Autodesk Fusion 360 part; units mm, degrees
sketch "Sketch1" plane through (0, 0, 0) normal (0, 0, 1) x (1, 0, 0)
  line L0 (-17.3001, 65.9212) -> (152.6999, 65.9212)
  line L1 (152.6999, 65.9212) -> (152.6999, -74.0788)
  line L2 (152.6999, -74.0788) -> (-17.3001, -74.0788)
  line L3 (-17.3001, -74.0788) -> (-17.3001, 65.9212)
  dimension "d1" = 140
  dimension "d2" = 170
extrude "Extrude1" add sketch "Sketch1" along normal blind 5
sketch "Sketch6" plane through (0, 0, 5) normal (0, 0, 1) x (-1, 0, 0)
  line L0 (17.3001, 74.0788) -> (-152.6999, 74.0788)
  line L1 (-152.6999, 74.0788) -> (-152.6999, -65.9212)
  line L2 (-152.6999, -65.9212) -> (17.3001, -65.9212)
  line L3 (17.3001, -65.9212) -> (17.3001, 74.0788)
  line L4 (-2.6999, 54.0788) -> (-132.6999, 54.0788)
  line L5 (-132.6999, 54.0788) -> (-132.6999, -45.9212)
  line L6 (-132.6999, -45.9212) -> (-2.6999, -45.9212)
  line L7 (-2.6999, -45.9212) -> (-2.6999, 54.0788)
  line L8 (17.3001, 74.0788) -> (17.3001, -65.9212)
  line L9 (-152.6999, -65.9212) -> (-152.6999, 74.0788)
  line L10 (-152.6999, 74.0788) -> (17.3001, 74.0788)
  line L11 (17.3001, -65.9212) -> (-152.6999, -65.9212)
  line L12 (-2.6999, 54.0788) -> (-12.6999, 54.0788)
  line L13 (-12.6999, 54.0788) -> (-12.6999, 44.0788)
  line L14 (-12.6999, 44.0788) -> (-2.6999, 44.0788)
  line L15 (-2.6999, 44.0788) -> (-2.6999, 54.0788)
  line L16 (-2.6999, -45.9212) -> (-12.6999, -45.9212)
  line L17 (-12.6999, -45.9212) -> (-12.6999, -35.9212)
  line L18 (-12.6999, -35.9212) -> (-2.6999, -35.9212)
  line L19 (-2.6999, -35.9212) -> (-2.6999, -45.9212)
  line L20 (-132.6999, 54.0788) -> (-122.6999, 54.0788)
  line L21 (-122.6999, 54.0788) -> (-122.6999, 44.0788)
  line L22 (-122.6999, 44.0788) -> (-132.6999, 44.0788)
  line L23 (-132.6999, 44.0788) -> (-132.6999, 54.0788)
  line L24 (-132.6999, -45.9212) -> (-122.6999, -45.9212)
  line L25 (-122.6999, -45.9212) -> (-122.6999, -35.9212)
  line L26 (-122.6999, -35.9212) -> (-132.6999, -35.9212)
  line L27 (-132.6999, -35.9212) -> (-132.6999, -45.9212)
  line L28 (-62.6999, 54.0788) -> (-72.6999, 54.0788)
  line L29 (-72.6999, 54.0788) -> (-72.6999, 44.0788)
  line L30 (-72.6999, 44.0788) -> (-62.6999, 44.0788)
  line L31 (-62.6999, 44.0788) -> (-62.6999, 54.0788)
  line L32 (-62.6999, -45.9212) -> (-72.6999, -45.9212)
  line L33 (-72.6999, -45.9212) -> (-72.6999, -35.9212)
  line L34 (-72.6999, -35.9212) -> (-62.6999, -35.9212)
  line L35 (-62.6999, -35.9212) -> (-62.6999, -45.9212)
  line L36 (-22.6999, -25.9212) -> (-112.6999, -25.9212)
  line L37 (-112.6999, -25.9212) -> (-112.6999, 34.0788)
  line L38 (-112.6999, 34.0788) -> (-22.6999, 34.0788)
  line L39 (-22.6999, 34.0788) -> (-22.6999, -25.9212)
  dimension "d23" = 20
  dimension "d24" = 20
  dimension "d25" = 20
  dimension "d26" = 20
  dimension "d27" = 10
  dimension "d28" = 10
  dimension "d29" = 10
  dimension "d30" = 10
  dimension "d31" = 10
  dimension "d32" = 10
  dimension "d33" = 10
  dimension "d34" = 10
  dimension "d35" = 10
  dimension "d36" = 10
  dimension "d37" = 10
  dimension "d38" = 10
  dimension "d39" = 50
  dimension "d40" = 50
  dimension "d41" = 50
  dimension "d42" = 50
  dimension "d57" = 10
  dimension "d58" = 10
  dimension "d59" = 10
  dimension "d60" = 10
  dimension "d61" = 20
  dimension "d62" = 20
extrude "Extrude4" add sketch "Sketch6" along normal blind 105 contours L4 L7 L12 L13 L14 L15 | L4 L28 L29 L30 L31 | L6 L7 L16 L17 L18 L19 | L4 L5 L20 L21 L22 L23 | L6 L32 L33 L34 L35 | L5 L6 L24 L25 L26 L27
sketch "Sketch7" plane through (0, 0, 110) normal (0, 0, 1) x (-1, 0, 0)
  line L0 (-2.6999, 44.0788) -> (-2.6999, 54.0788)
  line L1 (-2.6999, 54.0788) -> (-12.6999, 54.0788)
  line L2 (-12.6999, 54.0788) -> (-12.6999, 44.0788)
  line L3 (-12.6999, 44.0788) -> (-2.6999, 44.0788)
  line L4 (-2.6999, 54.0788) -> (-132.6999, 54.0788)
  line L5 (-132.6999, 54.0788) -> (-132.6999, -45.9212)
  line L6 (-132.6999, -45.9212) -> (-2.6999, -45.9212)
  line L7 (-2.6999, -45.9212) -> (-2.6999, 54.0788)
  dimension "d45" = 130
  dimension "d46" = 100
extrude "Extrude5" add sketch "Sketch7" along normal blind 5
sketch "Sketch8" plane through (0, 0, 115) normal (0, 0, 1) x (-1, 0, 0)
  line L0 (-2.6999, -45.9212) -> (-2.6999, 54.0788)
  line L1 (-2.6999, 54.0788) -> (-132.6999, 54.0788)
  line L2 (-132.6999, 54.0788) -> (-132.6999, -45.9212)
  line L3 (-132.6999, -45.9212) -> (-2.6999, -45.9212)
  line L4 (-57.6999, -15.9212) -> (-77.6999, -15.9212)
  line L5 (-77.6999, -15.9212) -> (-77.6999, 24.0788)
  line L6 (-77.6999, 24.0788) -> (-57.6999, 24.0788)
  line L7 (-57.6999, 24.0788) -> (-57.6999, -15.9212)
  dimension "d49" = 40
  dimension "d50" = 20
  dimension "d51" = 55
  dimension "d52" = 55
  dimension "d53" = 30
  dimension "d54" = 30
extrude "Extrude6" add sketch "Sketch8" along normal blind 5 contours L4 L5 L6 L7
extrude "Extrude7" cut sketch "Sketch6" against normal blind 5 contours L36 L37 L38 L39
Geometry: final body of the model. Coordinates: model frame, mm. A direction names the side the tool comes from. Give positions to 0.01 mm unless a question says otherwise; leave off trailing zeros. Order: outer loops, then holes, each group sorted by start corner. A loop starts at its lowest first (then second) coordinate and runs counter-clockwise, first axis right, second up. Notation, with made-up numbers: (9.25, -0.75) -> (30.25, -0.75) arc R22 ccw to (30.25, 31.25) -> close; hole circle Ø11 at (27, -15.75). An arc over 180 degrees is marked (long way). Write each question's results on one line, items separated by ' | '. Start each with the question number.
1) Section D-D (y = -21.5). Return loops of the section in (x, z), then the cut area to 3 significant figures.
2) First-contact query: pin 1 (3 mm diameter, centred on y = 43, z = 105, fed in from -X); pin 2 (8 mm diameter, centred on y = 43, z = 53, fed in from +X); pin 3 (3 mm diameter, centred on x = 129, z = 50, fed in from +Y). Flat tips, straight axial feed; report the tip coordinate or a pass-through.
3) Section A-A (y = -37.5). Return loops of the section in (x, z), then the cut area to 3 significant figures.
4) Draft query along Z for faces 1 (the flat face through (72.7, -49, 57)), 2 (the flat face through (57.7, -4, 117)), 3 (the flat face through (67, 28, 0)), 4 (the flat face through (62.7, -49, 57)). Return one class per face: pulls with the +Z half, pulls with the -Z half, needs draft (parallel to the pull), parting line crosses it, or undercut.
5) Set-up query: faces 5 (the flat face through (132.7, -45, 68)), 6 (the flat face through (22.7, -4, 3)), 7 (the flat face through (68, 45.921, 64)). Return all of +Z, -Z, +X, -X, +Y, -Y with unobstructed straight access to the full face (end or side cutting, diameter ignored); none if empty.
6) Section B-B (z = 22). Return loops of the section in (x, y), then the cut area to 3 significant figures.
7) Section C-C (x = 17.5). Return loops of the section in (y, z), then the cut area to 3 significant figures.
8) Line query: line 1 (X direction, y = 45, z = 94.5); line 2 (Z direction, x = 103, y = -46); line 3 (Y direction, x = 8.5, z = 101.5). Output: solid intervals per line, ascending. Write a range as from..to.
Calculated:
1) outline: (-17.3, 0) -> (22.7, 0) -> (22.7, 5) -> (-17.3, 5) -> close; (2.7, 110) -> (132.7, 110) -> (132.7, 115) -> (77.7, 115) -> (77.7, 120) -> (57.7, 120) -> (57.7, 115) -> (2.7, 115) -> close; (112.7, 0) -> (152.7, 0) -> (152.7, 5) -> (112.7, 5) -> close | area: 1,150 mm2
2) pin 1: x = 2.7 | pin 2: x = 132.7 | pin 3: y = 45.92
3) outline: (-17.3, 0) -> (152.7, 0) -> (152.7, 5) -> (-17.3, 5) -> close; (2.7, 110) -> (132.7, 110) -> (132.7, 115) -> (2.7, 115) -> close | area: 1,500 mm2
4) face 1: undercut | face 2: needs draft | face 3: pulls with the -Z half | face 4: undercut
5) face 5: +Z, +X, +Y, -Y | face 6: -Z | face 7: +Z, +X, -X, +Y
6) outline: (2.7, -54.08) -> (12.7, -54.08) -> (12.7, -44.08) -> (2.7, -44.08) -> close; (2.7, 35.92) -> (12.7, 35.92) -> (12.7, 45.92) -> (2.7, 45.92) -> close; (62.7, -54.08) -> (72.7, -54.08) -> (72.7, -44.08) -> (62.7, -44.08) -> close; (62.7, 35.92) -> (72.7, 35.92) -> (72.7, 45.92) -> (62.7, 45.92) -> close; (122.7, -54.08) -> (132.7, -54.08) -> (132.7, -44.08) -> (122.7, -44.08) -> close; (122.7, 35.92) -> (132.7, 35.92) -> (132.7, 45.92) -> (122.7, 45.92) -> close | area: 600 mm2
7) outline: (-74.08, 0) -> (65.92, 0) -> (65.92, 5) -> (-74.08, 5) -> close; (-54.08, 110) -> (45.92, 110) -> (45.92, 115) -> (-54.08, 115) -> close | area: 1,200 mm2
8) line 1: 2.7..12.7, 62.7..72.7, 122.7..132.7 | line 2: 0..5, 110..115 | line 3: -54.08..-44.08, 35.92..45.92
